Design review of the part shown in the three views and the two pictorial views. Dimensions are in mm from the part's minimum x, y and z. Coordinates: 2 decimals unless noted, no trailing zeros. Loops run counter-clockwise (first coordinate to the right, second up) from the corner with the lowest first, then second, coordinate; pieces in that order, holes last. Notation, with made-up numbers: (-8, -39.75) -> (33, -39.75) arc R31 cw to (33, -3.75) -> close; hole circle Ø10 at (3, 43). An arc over 180 degrees is marked (long way). One line per item, written item: value.
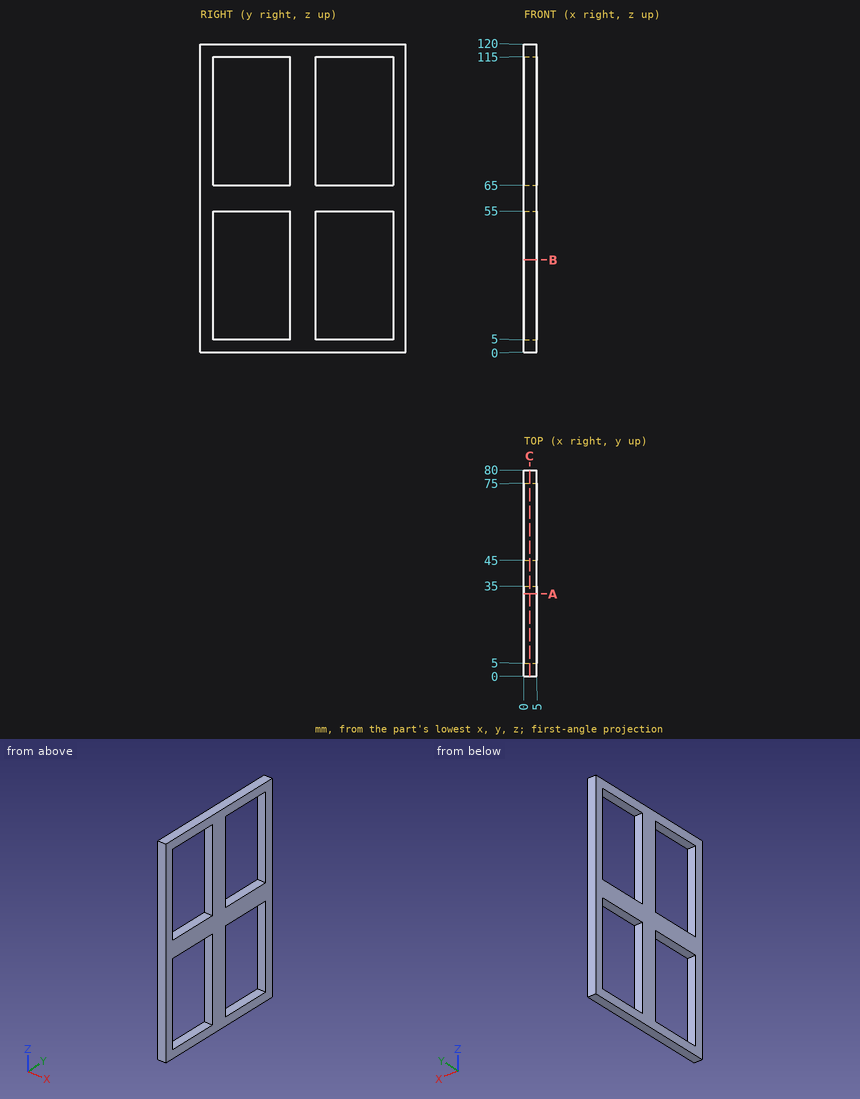
1. Take a section at B-B, the plane z = 36. Give the boundary of the cut face in (x, y).
Return value:
outline: (0, 0) -> (5, 0) -> (5, 5) -> (0, 5) -> close; (0, 35) -> (5, 35) -> (5, 45) -> (0, 45) -> close; (0, 75) -> (5, 75) -> (5, 80) -> (0, 80) -> close
2. Take a section at A-A, the plane y = 32. Give the boundary of the cut face in (x, z).
Return value:
outline: (0, 0) -> (5, 0) -> (5, 5) -> (0, 5) -> close; (0, 55) -> (5, 55) -> (5, 65) -> (0, 65) -> close; (0, 115) -> (5, 115) -> (5, 120) -> (0, 120) -> close
3. To check wall thickness, follow probe 1 along Y at (x, z) = (0.5, 49); probe 2 along Z at (x, y) = (3.7, 27.5). State the ranges of each line that lie inside material, in increasing order. Write a range as from..to.
Return value:
probe 1: y = 0..5, 35..45, 75..80
probe 2: z = 0..5, 55..65, 115..120
4. Take a section at C-C, the plane x = 2.2. Give the boundary of the cut face in (y, z).
Return value:
outline: (0, 0) -> (80, 0) -> (80, 120) -> (0, 120) -> close; hole (5, 5) -> (35, 5) -> (35, 55) -> (5, 55) -> close; hole (5, 65) -> (35, 65) -> (35, 115) -> (5, 115) -> close; hole (45, 5) -> (75, 5) -> (75, 55) -> (45, 55) -> close; hole (45, 65) -> (75, 65) -> (75, 115) -> (45, 115) -> close
